```python
from build123d import *

# Parameters (mm, degrees)
F1_DEPTH = 2.54
F3_DEPTH = 2.54


with BuildPart() as f1:
    # F0 (on Top) → F1 (new body)
    with BuildSketch(Plane.XY):
        with BuildLine():
            ThreePointArc((-16.51, 38.1), (-6.466491, 0.406925), (-12.7, -38.1))
            Line((-12.7, -38.1), (-6.35, -38.1))
            Line((-6.35, -38.1), (-6.35, -41.275))
            Line((-6.35, -41.275), (6.35, -41.275))
            Line((6.35, -41.275), (6.35, -38.1))
            Line((6.35, -38.1), (12.7, -38.1))
            ThreePointArc((12.7, -38.1), (6.466491, 0.406925), (16.51, 38.1))
            Line((16.51, 38.1), (6.35, 38.1))
            Line((6.35, 38.1), (6.35, 41.275))
            Line((6.35, 41.275), (-6.35, 41.275))
            Line((-6.35, 41.275), (-6.35, 38.1))
            Line((-6.35, 38.1), (-16.51, 38.1))
        make_face()
    extrude(amount=F1_DEPTH)

    # F2 (on face) → F3 (cut, through all)
    with BuildSketch(Plane.XY.offset(2.54)):
        with BuildLine():
            ThreePointArc((-10.511564, 34.29), (-2.646525, 0.293267), (-7.297803, -34.29))
            Line((-7.297803, -34.29), (7.297803, -34.29))
            ThreePointArc((7.297803, -34.29), (2.646525, 0.293267), (10.511564, 34.29))
            Line((10.511564, 34.29), (-10.511564, 34.29))
        make_face()
    extrude(amount=-F3_DEPTH, mode=Mode.SUBTRACT)


solid = f1.part
```
Input: part model. Units: mm. Frame: model coordinates. A direction names the side the tool comes from. Give positions to 0.01 mm unless a question says otherwise; leave off trailing zeros. Order: outer loops, then holes, each group sorted by start corner. A loop starts at its lowest first (then second) coordinate and runs counter-clockwise, first axis right, second up.
1. Line query: probe 1 along X at (y, z) = (1, 0.95); probe 2 along Y at (x, z) = (-1.5, 0.7) (3 decimals); probe 3 along X at (y, z) = (27, 1.85). Output: solid intervals per line, ascending.
Computed:
probe 1: x = -6.5 to -2.68, 2.68 to 6.5
probe 2: y = -41.275 to -34.29, 34.29 to 41.275
probe 3: x = -11.74 to -7.7, 7.7 to 11.74
2. Cut plane B-B (z = 1.65). Return loops of the section in (x, y) (3 decimals), and give its area (3 significant figures).
Computed:
outline: (-16.51, 38.1) arc R93.367 cw to (-12.7, -38.1) - (-6.35, -38.1) - (-6.35, -41.275) - (6.35, -41.275) - (6.35, -38.1) - (12.7, -38.1) arc R93.367 cw to (16.51, 38.1) - (6.35, 38.1) - (6.35, 41.275) - (-6.35, 41.275) - (-6.35, 38.1) - close; hole (-10.512, 34.29) arc R97.177 cw to (-7.298, -34.29) - (7.298, -34.29) arc R97.177 cw to (10.512, 34.29) - close
area: 826 mm2
3. Cut plane A-A (x = -1.5). Return loops of the section in (y, z) (3 decimals).
Computed:
outline: (-41.275, 0) - (-34.29, 0) - (-34.29, 2.54) - (-41.275, 2.54) - close; (34.29, 0) - (41.275, 0) - (41.275, 2.54) - (34.29, 2.54) - close
4. Draft query along Y for faces 4 (the face through (-6.5, 1, 1.3)), 5 (the face through (12, 38.1, 1)), 6 (the face through (9, -38.1, 1)). Return one class per face: released by +Y, released by -Y, zero draft, split by the parting line, or undercut.
Computed:
face 4: undercut
face 5: released by +Y
face 6: released by -Y
5. Set-up query: faces 1 (the face through (6.35, 40, 1)), 2 (the face through (6.35, -40, 1)), 3 (the face through (-6.35, 40, 1)). Return all of +Z, -Z, +X, -X, +Y, -Y with unobstructed straight access to the full face (end or side cutting, diameter ignored); none if empty.
Computed:
face 1: +Z, -Z, +X, +Y
face 2: +Z, -Z, +X, -Y
face 3: +Z, -Z, -X, +Y
6. Cut plane C-C (y = 13.5). Return loops of the section in (x, z).
Computed:
outline: (-8.05, 0) - (-4.18, 0) - (-4.18, 2.54) - (-8.05, 2.54) - close; (4.18, 0) - (8.05, 0) - (8.05, 2.54) - (4.18, 2.54) - close
7. Pin query (flat end, axial travel): pin 1 Ø0.8 at (x, z) = (9, 1.5) entering from +Y; pin 2 Ø1.5 at (y, z) = (27.5, 2) entering from -X; pin 3 Ø1.3 at (y, z) = (40.5, 1.5) entering from -X. Return the tip coordinate at first contact, or that it passes through.
Computed:
pin 1: stops at y = 38.1
pin 2: stops at x = -12.19
pin 3: stops at x = -6.35
